Check sheet for the modelled part. Datum: model origin and axes. Units: mm. A direction names the side the tool comes from. Coordinates: 2 decimals unless noted, no trailing zeros. Loops run counter-clockwise (first coordinate to the right, second up) from the corner with the lowest first, then second, coordinate; pieces in that order, holes last. Notation, with made-up numbers: M 59.25,-22 L 99.25,-22 A5 ccw 99.25,-13 Z; hole C 76,-23.75 d3. An arc over 180 degrees is marked long. Write each question's results on one line, items separated by ' | '. Start each with the question number.
from build123d import *

# Parameters (mm, degrees)
ESQUISSE1_W             = 6.35
ESQUISSE1_H             = 5.97
BOSS_EXTRU_1_DEPTH      = 2.19
CHANFREIN1_SIZE         = 0.8
CHANFREIN1_SIZE2        = 0.5
CHANFREIN2_SIZE         = 0.5
CHANFREIN2_SIZE2        = 0.8
CHANFREIN3_SIZE         = 0.8
CHANFREIN3_SIZE2        = 0.5
CHANFREIN4_SIZE         = 0.5
CHANFREIN4_SIZE2        = 0.8
CHANFREIN5_SIZE         = 0.8
CHANFREIN5_SIZE2        = 0.5
CHANFREIN6_SIZE         = 0.5
CHANFREIN6_SIZE2        = 0.8
CHANFREIN7_SIZE         = 2
CHANFREIN7_SIZE2        = 0.5
ESQUISSE2_W             = 5
ESQUISSE2_H             = 0.65
BOSS_EXTRU_2_DEPTH      = 1.27
BOSS_EXTRU_2_DEPTH_BACK = 5
CHANFREIN8_SIZE         = 0.5


with BuildPart() as part:
    # Esquisse1 → Boss.-Extru.1 (new body)
    with BuildSketch(Plane.XY):
        with Locations((3.175, 2.985)):
            Rectangle(ESQUISSE1_W, ESQUISSE1_H)
    extrude(amount=BOSS_EXTRU_1_DEPTH)

    # Chanfrein1
    chanfrein1_edges = [part.edges().sort_by_distance(p)[0] for p in [
        (6.35, 2.985, 2.19),
    ]]
    chanfrein1_side = [part.faces().sort_by_distance(p)[0] for p in [
        (6.35, 2.985, 1.095),
    ]]
    chamfer(chanfrein1_edges, length=CHANFREIN1_SIZE, length2=CHANFREIN1_SIZE2, reference=chanfrein1_side[0])

    # Chanfrein2
    chanfrein2_edges = [part.edges().sort_by_distance(p)[0] for p in [
        (6.35, 2.985, 0),
    ]]
    chanfrein2_side = [part.faces().sort_by_distance(p)[0] for p in [
        (3.175, 2.985, 0),
    ]]
    chamfer(chanfrein2_edges, length=CHANFREIN2_SIZE, length2=CHANFREIN2_SIZE2, reference=chanfrein2_side[0])

    # Chanfrein3
    chanfrein3_edges = [part.edges().sort_by_distance(p)[0] for p in [
        (2.925, 0, 2.19),
    ]]
    chanfrein3_side = [part.faces().sort_by_distance(p)[0] for p in [
        (3.085907094, 0, 1.095),
    ]]
    chamfer(chanfrein3_edges, length=CHANFREIN3_SIZE, length2=CHANFREIN3_SIZE2, reference=chanfrein3_side[0])

    # Chanfrein4
    chanfrein4_edges = [part.edges().sort_by_distance(p)[0] for p in [
        (2.925, 0, 0),
    ]]
    chanfrein4_side = [part.faces().sort_by_distance(p)[0] for p in [
        (2.925, 2.985, 0),
    ]]
    chamfer(chanfrein4_edges, length=CHANFREIN4_SIZE, length2=CHANFREIN4_SIZE2, reference=chanfrein4_side[0])

    # Chanfrein5
    chanfrein5_edges = [part.edges().sort_by_distance(p)[0] for p in [
        (0, 3.235, 2.19),
    ]]
    chanfrein5_side = [part.faces().sort_by_distance(p)[0] for p in [
        (0, 3.073946398, 1.095),
    ]]
    chamfer(chanfrein5_edges, length=CHANFREIN5_SIZE, length2=CHANFREIN5_SIZE2, reference=chanfrein5_side[0])

    # Chanfrein6
    chanfrein6_edges = [part.edges().sort_by_distance(p)[0] for p in [
        (0, 3.235, 0),
    ]]
    chanfrein6_side = [part.faces().sort_by_distance(p)[0] for p in [
        (2.925, 3.235, 0),
    ]]
    chamfer(chanfrein6_edges, length=CHANFREIN6_SIZE, length2=CHANFREIN6_SIZE2, reference=chanfrein6_side[0])

    # Chanfrein7
    chanfrein7_edges = [part.edges().sort_by_distance(p)[0] for p in [
        (3.175, 5.97, 2.19),
    ]]
    chanfrein7_side = [part.faces().sort_by_distance(p)[0] for p in [
        (3.175, 5.97, 1.095),
    ]]
    chamfer(chanfrein7_edges, length=CHANFREIN7_SIZE, length2=CHANFREIN7_SIZE2, reference=chanfrein7_side[0])

    # Esquisse2 → Boss.-Extru.2 (add, two sides)
    with BuildSketch(Plane(origin=(0, 5.97, 0), x_dir=(-1, 0, 0), z_dir=(0, 1, 0))) as boss_extru_2_sk:
        with Locations((-3.175, 0.325)):
            Rectangle(ESQUISSE2_W, ESQUISSE2_H)
    extrude(amount=BOSS_EXTRU_2_DEPTH)
    extrude(boss_extru_2_sk.sketch, amount=-BOSS_EXTRU_2_DEPTH_BACK)

    # Chanfrein8
    chanfrein8_edges = [part.edges().sort_by_distance(p)[0] for p in [
        (0.675, 7.24, 0.325),
        (5.675, 7.24, 0.325),
    ]]
    chamfer(chanfrein8_edges, length=CHANFREIN8_SIZE)


solid = part.part
1) Set-up check for faces 1 (the flat face through (6.096, 2.795, 1.796)), 2 (the flat face through (3, 7, 0.65)): record each of +Z, -Z, +X, -X, +Y, -Y from which the full face is reachable in a straight line by a thin tool's end or side.
2) Section check C-C (y = 3.5). Enter the section's corners in (x, z), then the cut area to 3 significant figures.
3) Gauge pin test, flat end, axial feed: P1, Ø0.5, axis at y = 6.5, z = 0.5, coming from the -X side (3 decimals). Record the tip position at first contact, or that the pin passes through.
4) Section check D-D (z = 0.9). Enter the section's corners in (x, y), then the cut area to 3 significant figures.
5) Thickness scan on probe 1 along X at (y, z) = (6, 0.6) (3 decimals); probe 2 along X at (y, z) = (5.25, 2); probe 3 along Y at (x, z) = (5.75, 0.5). Record the ranges inside material, lowest first.
6) Section check B-B (z = 0.35). Enter the section's corners in (x, y) (3 decimals).
7) Section check A-A (x = 4.5). Enter the section's corners in (y, z) (3 decimals).
Return value:
1) face 1: +Z, +X, +Y, -Y | face 2: +Z, +X, -X, +Y
2) outline: M 0,0.8 L 0.5,0 L 5.85,0 L 6.35,0.8 L 6.35,1.39 L 5.85,2.19 L 0.5,2.19 L 0,1.39 Z | area: 13.1 mm2
3) P1: stops at x = 0.675
4) outline: M 0,0 L 6.35,0 L 6.35,5.79 L 0,5.79 Z | area: 36.8 mm2
5) probe 1: x = 0.675 to 5.675 | probe 2: x = 0.38 to 5.97 | probe 3: y = 0.19 to 5.89
6) outline: M 0.281,0.281 L 6.069,0.281 L 6.069,5.93 L 5.675,5.93 L 5.675,6.74 L 5.175,7.24 L 1.175,7.24 L 0.675,6.74 L 0.675,5.93 L 0.281,5.93 Z
7) outline: M 0,0.8 L 0.5,0 L 7.24,0 L 7.24,0.65 L 5.855,0.65 L 5.47,2.19 L 0.5,2.19 L 0,1.39 Z
